The figure shows three views and two pictorial views of one solid part (mm, origin at its lowest corner). Answer the questions. A direction names the side the tool comes from. Give positions to 0.01 mm unless a question says otherwise; leave off trailing zeros. Write each loop counter-clockwise with the first axis right and the second up, starting at its lowest first coordinate (ties: lowest second). Pieces come first, ordered by that corner, then holes. Notation, with made-up numbers: (45, 56.5) - (77, 56.5) arc R13 ccw to (77, 75.5) - close; hole circle Ø8 at (-6, 39). An arc over 180 degrees is marked (long way). Answer as CSV lines item,"result". Start each with the question number.
(1) For the marked faces 1 and 2, determine the directions among +Z, -Z, +X, -X, +Y, -Y from which every point of the face is accessible in a straight line to the end or side of a thin tool.
(2) Find section D-D (z = 15.5). Write down the section's boundary in (x, y), then the cut area to 3 significant figures.
(3) Straight lines are drawn through the part: probe 1 along Z at (x, y) = (81.5, 1.5) (1 decimal); probe 2 along X at (y, z) = (3.75, 73); probe 3 along Z at (x, y) = (102, 4.75) (1 decimal). For each, find the intervals that lie inside material, in ascending order.
(4) Find section A-A (x = 62.5). Write down the section's boundary in (y, z).
(5) For a pull along Z with two mould halves and no side action, classify the marked faces 3 and 4 as pulls with the +Z half, pulls with the -Z half, needs draft (parallel to the pull), parting line crosses it, or undercut.
(6) Find section B-B (z = 100). Write down the section's boundary in (x, y).
(7) Find section C-C (y = 2.5). State how many separate pieces and enclosed holes the cut face has, then the cut area to 3 significant figures.
(8) Each of these flat-tipped pins is pushed along its axis until it touches: pin 1 Ø4 at (y, z) = (2, 70) entering from -X; pin 2 Ø18 at (x, z) = (41.5, 32.5) entering from -Y; pin 3 Ø2 at (y, z) = (4, 20.5) entering from +X. Where does it stop, or does it pass through?
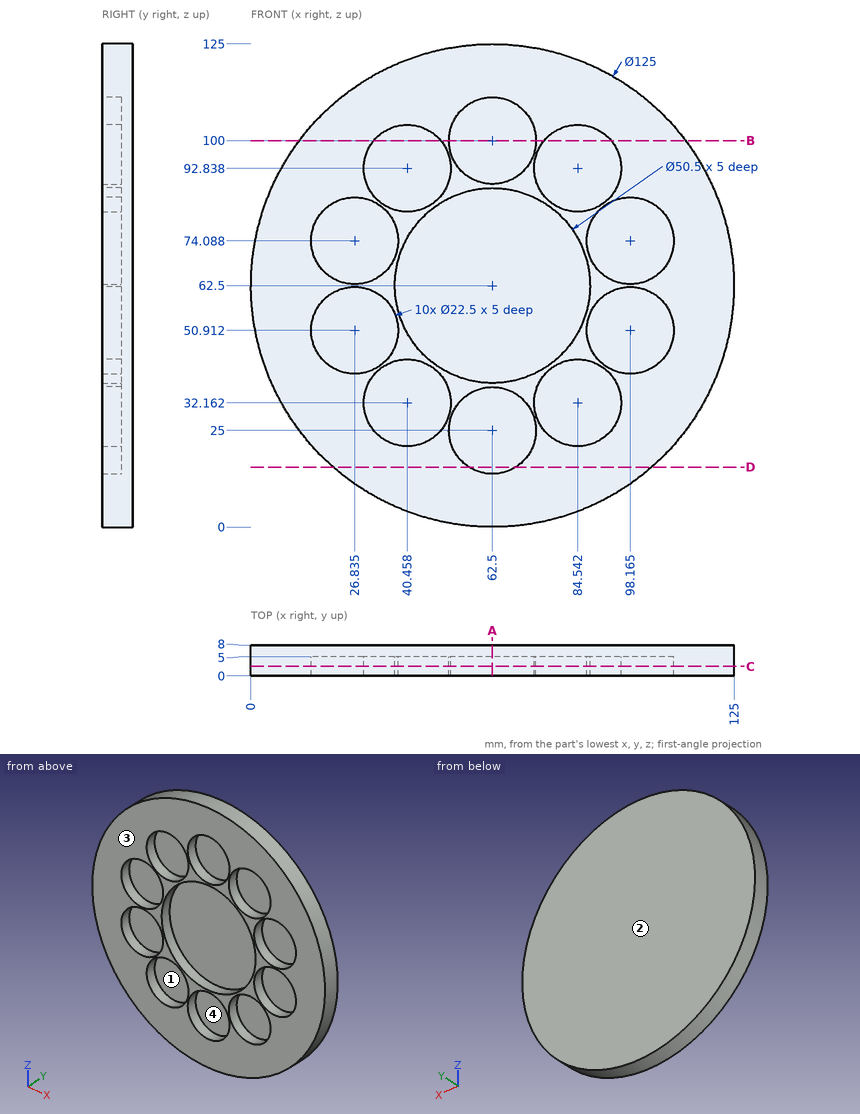
Result set:
1,face 1,"-Y"
1,face 2,"+Z, -Z, +X, -X, +Y"
2,outline,"(21.3, 0) - (56.47, 0) - (56.47, 5) - (68.53, 5) - (68.53, 0) - (103.7, 0) - (103.7, 8) - (21.3, 8) - close"
2,area,"599 mm^2"
3,probe 1,"3 to 21.3, 43 to 45.9, 79.1 to 82, 103.7 to 122"
3,probe 2,"0.89 to 15.64, 38.03 to 39.54, 85.46 to 86.97, 109.36 to 124.11"
3,probe 3,"14.1 to 40.3, 61.5 to 63.5, 84.7 to 110.9"
4,outline,"(0, 0) - (8, 0) - (8, 125) - (0, 125) - (0, 111.25) - (5, 111.25) - (5, 88.75) - (0, 88.75) - (0, 87.75) - (5, 87.75) - (5, 37.25) - (0, 37.25) - (0, 36.25) - (5, 36.25) - (5, 13.75) - (0, 13.75) - close"
5,face 3,"needs draft"
5,face 4,"undercut"
6,outline,"(12.5, 0) - (31.78, 0) - (31.78, 5) - (49.13, 5) - (49.13, 0) - (51.25, 0) - (51.25, 5) - (73.75, 5) - (73.75, 0) - (75.87, 0) - (75.87, 5) - (93.22, 5) - (93.22, 0) - (112.5, 0) - (112.5, 8) - (12.5, 8) - close"
7,separate pieces,"1"
7,enclosed holes,"11"
7,area,"6,290 mm^2"
8,pin 1,"x = 0.24"
8,pin 2,"y = 5"
8,pin 3,"x = 109.67"
